Check sheet for the drawn part. Datum: minimum x, y, z corner. Units: mm. A direction names the side the tool comes from. Give positions to 0.01 mm unless a question says otherwise; leave off trailing zeros. Write each loop counter-clockwise with the first axis right and the second up, starting at its lowest first coordinate (ties: lowest second). Pieces come first, ordered by that corner, then holes. Notation, with made-up numbers: (-39.5, 48) - (-27.5, 48) arc R31 ccw to (-27.5, 76) - close; hole circle Ø8 at (-18.5, 22.5). An arc over 180 degrees is marked (long way). Use a Markdown table: item, result.
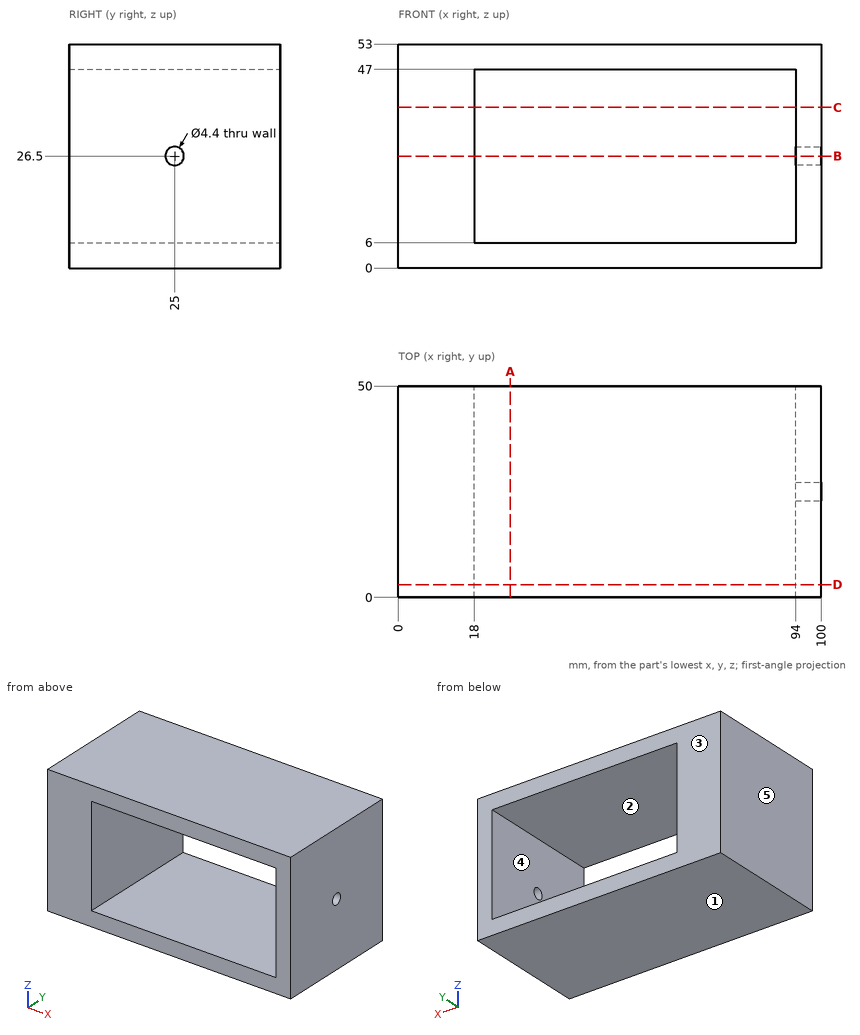
1) Section check A-A on x = 26.5. Record the boundary of the cut face in (y, z).
Working result:
| item | result |
|---|---|
| outline | (0, 0) - (50, 0) - (50, 6) - (0, 6) - close; (0, 47) - (50, 47) - (50, 53) - (0, 53) - close |
2) Section check C-C on z = 38. Record the boundary of the cut face in (x, y).
Working result:
| item | result |
|---|---|
| outline | (0, 0) - (18, 0) - (18, 50) - (0, 50) - close; (94, 0) - (100, 0) - (100, 50) - (94, 50) - close |
3) Material ranges on L1, parallel to X at y = 6, z = 7.5; L2, parallel to Z at x = 36.5, y = 35; L3, parallel to Y at x = 98.8, z = 26.5, recorded low to high. Write a range as from..to.
Working result:
| item | result |
|---|---|
| L1 | x = 0..18, 94..100 |
| L2 | z = 0..6, 47..53 |
| L3 | y = 0..22.8, 27.2..50 |
4) Mould release check, pull along Z, two halves, no side actions. Record for the marked faces 1, 2 and 3: pulls with the +Z half, pulls with the -Z half, needs draft (parallel to the pull), parting line crosses it, or undercut.
Working result:
| item | result |
|---|---|
| face 1 | pulls with the -Z half |
| face 2 | undercut |
| face 3 | needs draft |
5) Set-up check for the marked faces 4 and 5: record each of +Z, -Z, +X, -X, +Y, -Y from which the full face is reachable in a straight line by a thin tool's end or side.
Working result:
| item | result |
|---|---|
| face 4 | +Y, -Y |
| face 5 | +Z, -Z, -X, +Y, -Y |
6) Section check B-B on z = 26.5. Record the boundary of the cut face in (x, y), then the cut area to 3 significant figures.
Working result:
| item | result |
|---|---|
| outline | (0, 0) - (18, 0) - (18, 50) - (0, 50) - close; (94, 0) - (100, 0) - (100, 22.8) - (94, 22.8) - close; (94, 27.2) - (100, 27.2) - (100, 50) - (94, 50) - close |
| area | 1,170 mm² |
7) Depth check by flat-ended pin: P1, Ø10, axis at x = 25, z = 17.5, coming from the +Y side. Enter the tip coordinate at first touch or a pass-through.
Working result:
| item | result |
|---|---|
| P1 | passes through |
8) Section check D-D on y = 3. Record the boundary of the cut face in (x, z).
Working result:
| item | result |
|---|---|
| outline | (0, 0) - (100, 0) - (100, 53) - (0, 53) - close; hole (18, 6) - (94, 6) - (94, 47) - (18, 47) - close |
